Model file for the job. Use its own axes, mm. A direction names the side the tool comes from. Round coordinates to 2 decimals unless told otherwise and drop trailing zeros. Write each loop counter-clockwise with the first axis right and the second up, starting at its lowest first coordinate (ties: lowest second). Pieces come first, ordered by that corner, then holes.
```python
from build123d import *

# Parameters (mm, degrees)
SKETCH1_W           = 130
SKETCH1_H           = 136.666666666
SKETCH1_R           = 3.4
BOSS_EXTRUDE1_DEPTH = 5
SKETCH2_R           = 2.6
SKETCH2_W           = 70
SKETCH2_H           = 110.094716781
SKETCH2_W_2         = 5
SKETCH2_H_2         = 10
CUT_EXTRUDE1_DEPTH  = 5
FILLET1_R           = 5
FILLET2_R           = 1


with BuildPart() as part:
    # Sketch1 → Boss-Extrude1 (new body)
    with BuildSketch(Plane.XY):
        Rectangle(SKETCH1_W, SKETCH1_H)
        with Locations((-25, -43.333333333)):
            Circle(SKETCH1_R, mode=Mode.SUBTRACT)
        with Locations(Location((25, -43.333333333, 0), (0, 0, 180))):
            Circle(SKETCH1_R, mode=Mode.SUBTRACT)
    extrude(amount=BOSS_EXTRUDE1_DEPTH)

    # Sketch2 → Cut-Extrude1 (cut)
    with BuildSketch(Plane.XY.offset(5)):
        with Locations((-57.5, -45.833333333)):
            Circle(SKETCH2_R)
        with Locations(Location((57.5, -45.833333333, 0), (0, 0, 180))):
            Circle(SKETCH2_R)
        with Locations((0, 56.850465305)):
            Rectangle(SKETCH2_W, SKETCH2_H)
        with Locations((-57.5, -33.333333333)):
            Rectangle(SKETCH2_W_2, SKETCH2_H_2)
        with Locations((-57.5, -58.333333333)):
            Rectangle(SKETCH2_W_2, SKETCH2_H_2)
        with Locations((57.5, -33.333333333)):
            Rectangle(SKETCH2_W_2, SKETCH2_H_2)
        with Locations((57.5, -58.333333333)):
            Rectangle(SKETCH2_W_2, SKETCH2_H_2)
    extrude(amount=-CUT_EXTRUDE1_DEPTH, mode=Mode.SUBTRACT)

    # Fillet1
    fillet1_edges = [part.edges().sort_by_distance(p)[0] for p in [
        (35, 68.333333333, 2.5),
        (-35, 68.333333333, 2.5),
        (-35, 1.803106914, 2.5),
        (35, 1.803106914, 2.5),
        (-65, 68.333333333, 2.5),
        (65, 68.333333333, 2.5),
    ]]
    fillet(fillet1_edges, radius=FILLET1_R)

    # Fillet2
    fillet2_edges = [part.edges().sort_by_distance(p)[0] for p in [
        (65, -68.333333333, 2.5),
        (-65, -68.333333333, 2.5),
    ]]
    fillet(fillet2_edges, radius=FILLET2_R)


solid = part.part
```
1) Cut at B-B on x = -25. List the corners of the cut face in (y, z).
2) Wall check: probe 1 along Y at (x, z) = (-57.5, 2.75); probe 2 along Y at (x, z) = (-25, 2.4); probe 3 along X at (y, z) = (-36, 1.1). Give the ranges that are in metal, low to high.
3) Cut at A-A on x = -57.5. List the corners of the cut face in (y, z).
4) Pull direction X, two halves, no side cores. Call faces 4 (the face through (63.574, 66.83, 2.535)), 5 (the face through (-1, -68.333, 2)), 6 (the face through (0, 1.803, 3)), 7 (the face through (-65, -3, 2)): released by +X, released by -X, zero draft, split by the parting line, or undercut.
5) Cut at C-C on y = -58.5. List the corners of the cut face in (x, z).
6) Cut at D-D on x = -10.5. List the corners of the cut face in (y, z).
7) Which spindle directions (+Z, -Z, +X, -X, +Y, -Y) get a long thin tool onto all of the face, cutting with end or side? Do faces 1 (the face through (-55, -33, 3)), 2 (the face through (-36.504, 66.908, 2.465)), 3 (the face through (-50, 68.333, 2)). Say none if no direction does.
Result sheet:
1. outline: (-68.33, 0) - (-46.73, 0) - (-46.73, 5) - (-68.33, 5) - close; (-39.93, 0) - (1.8, 0) - (1.8, 5) - (-39.93, 5) - close
2. probe 1: y = -68.33 to -63.33, -53.33 to -48.43, -43.23 to -38.33, -28.33 to 68.33
2. probe 2: y = -68.33 to -46.73, -39.93 to 1.8
2. probe 3: x = -65 to -60, -55 to 55, 60 to 65
3. outline: (-68.33, 0) - (-63.33, 0) - (-63.33, 5) - (-68.33, 5) - close; (-53.33, 0) - (-48.43, 0) - (-48.43, 5) - (-53.33, 5) - close; (-43.23, 0) - (-38.33, 0) - (-38.33, 5) - (-43.23, 5) - close; (-28.33, 0) - (68.33, 0) - (68.33, 5) - (-28.33, 5) - close
4. face 4: released by +X
4. face 5: zero draft
4. face 6: undercut
4. face 7: released by -X
5. outline: (-65, 0) - (-60, 0) - (-60, 5) - (-65, 5) - close; (-55, 0) - (55, 0) - (55, 5) - (-55, 5) - close; (60, 0) - (65, 0) - (65, 5) - (60, 5) - close
6. outline: (-68.33, 0) - (1.8, 0) - (1.8, 5) - (-68.33, 5) - close
7. face 1: +Z, -Z
7. face 2: +Z, -Z, +Y
7. face 3: +Z, -Z, +X, -X, +Y
